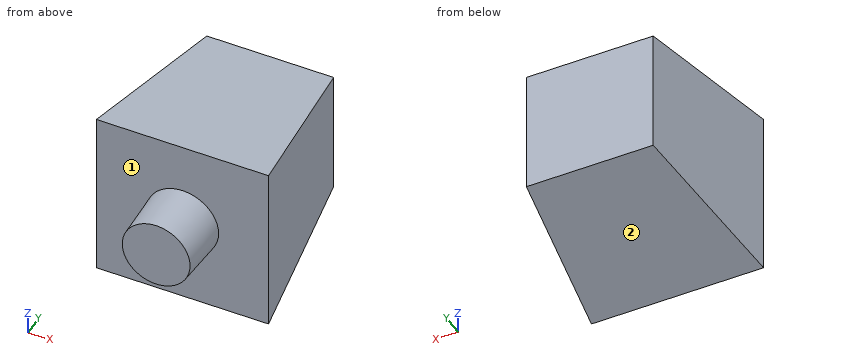
Autodesk Inventor part; units mm, degrees
ref_plane "YZ Plane" through (0, 0, 0) normal (1, 0, 0) x (0, 1, 0)
ref_plane "XZ Plane" through (0, 0, 0) normal (0, 1, 0) x (-1, 0, 0)
ref_plane "XY Plane" through (0, 0, 0) normal (0, 0, 1) x (1, 0, 0)
sketch "Sketch1" plane through (0, 0, 0) normal (0, 1, 0) x (-1, 0, 0)
  line L0 (0, 0) -> (10, 0)
  line L1 (10, 0) -> (10, -10)
  line L2 (10, -10) -> (0, -10)
  line L3 (0, -10) -> (0, 0)
  dimension "d0" = 10
  dimension "d1" = 10
extrude "Extrusion1" add sketch "Sketch1" along normal blind 10 draft -7.5
sketch "Sketch2" plane through (0, 0, 0) normal (0, -1, 0) x (1, 0, 0)
  circle A0 centre (-5, -5) radius 2.1
  line L0 (0, -10) -> (0, 0)
  line L1 (-10, -10) -> (0, -10)
  point P0 (0, -5)
  point P1 (-5, -10)
  dimension "d4" = 4.2
extrude "Extrusion2" add sketch "Sketch2" along normal blind 3 draft -2.5
properties part number "Press  Fit Foot A"
Input: part model. Units: mm. Frame: model coordinates. Face numbers are marked on the shaded views. A direction names the side the tool comes from. Give positions to 0.01 mm unless a question says otherwise; leave off trailing zeros. Order: outer loops, then holes, each group sorted by start corner. A loop starts at its lowest first (then second) coordinate and runs counter-clockwise, first axis right, second up. Notation, with made-up numbers: M 56.5,18.25 L 112.5,18.25 A11 cw 112.5,36.25 Z; hole C 10,4.5 d8. An arc over 180 degrees is marked long. Return JSON: item names as keys, results as strings.
1) Section query D-D on y = 4. Output: boundary loops of the cut face in (x, z), and give its area (3 significant figures).
Taken from the geometry:
{"outline": "M -9.47,-9.47 L -0.53,-9.47 L -0.53,-0.53 L -9.47,-0.53 Z", "area": "80.0 mm2"}
2) Section query A-A on z = -5. Output: boundary loops of the cut face in (x, y).
Taken from the geometry:
{"outline": "M -10,0 L -7.1,0 L -6.97,-3 L -3.03,-3 L -2.9,0 L 0,0 L -1.32,10 L -8.68,10 Z"}
3) Line query: L1, parallel to Y at x = -2.25, z = -5.5; L2, parallel to X at y = 4, z = -7.75; L3, parallel to X at y = 2.5, z = -5.5. Output: solid intervals per line, ascending. Write a range as [from, to].
Taken from the geometry:
{"L1": "y = [0, 10]", "L2": "x = [-9.47, -0.53]", "L3": "x = [-9.67, -0.33]"}
4) Access query for the marked faces 1 and 2. Directions: +Z, -Z, +X, -X, +Y, -Y. A direction counts if a zero-diameter tool reaches every point of the face in a straight line with its end or side. Return the directions, or none.
Taken from the geometry:
{"face 1": "-Y", "face 2": "-Z, +X, -X, +Y"}
5) Section query C-C on y = 7.75. Output: boundary loops of the cut face in (x, z).
Taken from the geometry:
{"outline": "M -8.98,-8.98 L -1.02,-8.98 L -1.02,-1.02 L -8.98,-1.02 Z"}
6) Section query B-B on x = -5. Output: boundary loops of the cut face in (y, z).
Taken from the geometry:
{"outline": "M -3,-6.97 L 0,-7.1 L 0,-10 L 10,-8.68 L 10,-1.32 L 0,0 L 0,-2.9 L -3,-3.03 Z"}
7) Contact query for a flat-ended pin moving along its axis: pin 1 (1 mm diameter, centred on y = 5.5, z = -6, fed in from -X). Output: stop coordinate, or through.
Taken from the geometry:
{"pin 1": "stops at x = -9.34"}
